For this review, take the finished solid that the model builds, in its own axes (mm). Give positions to 0.01 mm unless a question says otherwise; leave off trailing zeros. Loops run counter-clockwise (first coordinate to the right, second up) from the corner with the lowest first, then second, coordinate; pieces in that order, holes last. Notation, with made-up numbers: (23, 77.5) - (48, 77.5) arc R22 ccw to (48, 103.5) - close; hole circle Ø6 at (-12.75, -20.5). An arc over 180 degrees is marked (long way). Put each result on its own line as item: value.
Autodesk Inventor part; units mm, degrees
ref_plane "YZ Plane" through (0, 0, 0) normal (1, 0, 0) x (0, 1, 0)
ref_plane "XZ Plane" through (0, 0, 0) normal (0, 1, 0) x (-1, 0, 0)
ref_plane "XY Plane" through (0, 0, 0) normal (0, 0, 1) x (1, 0, 0)
sketch "Sketch1" plane through (0, 0, 0) normal (0, 1, 0) x (-1, 0, 0)
  line L0 (-47, 47) -> (47, 47)
  line L1 (47, 47) -> (47, -47)
  line L2 (47, -47) -> (-47, -47)
  line L3 (-47, -47) -> (-47, 47)
  line L4 (-47, 47) -> (47, -47) construction
  line L5 (47, 47) -> (-47, -47) construction
  line L6 (47, -35) -> (3, -35)
  line L7 (3, -35) -> (3, -47)
  line L8 (3, -47) -> (47, -47)
  line L9 (47, -47) -> (47, -35)
  line L10 (47, -3.667) -> (3, -3.667)
  line L11 (3, -3.667) -> (3, -27.667)
  line L12 (3, -27.667) -> (47, -27.667)
  line L13 (47, -27.667) -> (47, -3.667)
  point P0 (0, 0)
  point P1 (25, -47)
  point P2 (25, -35)
  dimension "d0" = 94
  dimension "d1" = 94
  dimension "d2" = 12
  dimension "d3" = 24
  dimension "d4" = 7.333
  dimension "d9" = 3
  dimension "d10" = 0
extrude "Extrusion1" add sketch "Sketch1" along normal blind 5
extrude "Extrusion2" cut sketch "Sketch1" along normal blind 5 contours L1 L12 L11 L10 | L7 L6 L1 L2
mirror "Mirror1" about plane through (0, 0, 0) normal (1, 0, 0) of "Extrusion2"
mirror "Mirror2" about plane through (0, 0, 0) normal (0, 0, 1) of "Extrusion2", "Mirror1"
properties part number "Grid RS3" material "Steel"
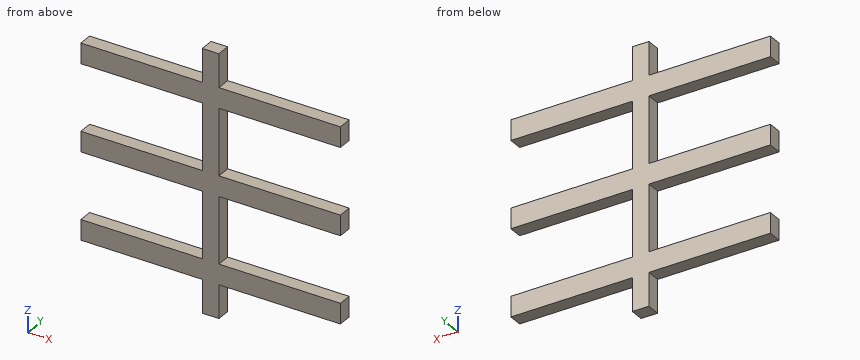
1) Take a section at B-B on y = 4.2. State the section outline as (x, z) points, and give its area (3 significant figures).
Geometry check:
outline: (-47, -35) - (-3, -35) - (-3, -47) - (3, -47) - (3, -35) - (47, -35) - (47, -27.67) - (3, -27.67) - (3, -3.67) - (47, -3.67) - (47, 3.67) - (3, 3.67) - (3, 27.67) - (47, 27.67) - (47, 35) - (3, 35) - (3, 47) - (-3, 47) - (-3, 35) - (-47, 35) - (-47, 27.67) - (-3, 27.67) - (-3, 3.67) - (-47, 3.67) - (-47, -3.67) - (-3, -3.67) - (-3, -27.67) - (-47, -27.67) - close
area: 2,500 mm²
2) Wall thickness on line 1 (Z direction, x = -8, y = 4.85); line 2 (X direction, y = 4.7, z = 17): over which ranges is each line inside the solid? List them lowest first.
Geometry check:
line 1: z = -35 to -27.67, -3.67 to 3.67, 27.67 to 35
line 2: x = -3 to 3
3) Insertion check: pin 1 Ø2.5 at (x, y) = (16, 2.5) entering from -Z; pin 2 Ø2.5 at (x, y) = (18.5, 2.5) entering from +Z; pin 3 Ø2.5 at (y, z) = (1.5, 42) entering from -X; pin 4 Ø10 at (x, z) = (3.5, -12) entering from +Y. Each pin has a flat end and moves straight along its axis. Give the tip position at first contact, or say it passes through.
Geometry check:
pin 1: stops at z = -35
pin 2: stops at z = 35
pin 3: stops at x = -3
pin 4: stops at y = 5
4) Take a section at C-C on z = -15.5. State the section outline as (x, y) points, and give its area (3 significant figures).
Geometry check:
outline: (-3, 0) - (3, 0) - (3, 5) - (-3, 5) - close
area: 30.0 mm²
5) Take a section at A-A on x = -35.5. State the section outline as (y, z) points.
Geometry check:
outline: (0, -35) - (5, -35) - (5, -27.67) - (0, -27.67) - close; (0, -3.67) - (5, -3.67) - (5, 3.67) - (0, 3.67) - close; (0, 27.67) - (5, 27.67) - (5, 35) - (0, 35) - close
